from build123d import *

# Parameters (mm, degrees)
BOSS_EXTRUDE1_DEPTH = 6.5
SKETCH2_OUTSIDE_W   = 43.518
SKETCH2_OUTSIDE_H   = 43.054
SKETCH2_OUTSIDE_R   = 6.5
CUT_EXTRUDE1_DEPTH  = 6.5
CUT_EXTRUDE1_DRAFT  = -60
SKETCH3_OUTSIDE_W   = 43.518
SKETCH3_OUTSIDE_H   = 43.054
SKETCH3_OUTSIDE_R   = 6.5
CUT_EXTRUDE2_DEPTH  = 6.5
CUT_EXTRUDE2_DRAFT  = -60
SKETCH4_R           = 4.5
CUT_EXTRUDE3_DEPTH  = 13.125271319


with BuildPart() as part:
    # Sketch1 → Boss-Extrude1 (new body)
    with BuildSketch(Plane.XY):
        Polygon((4.981175881, 5.614376205), (-2.371604479, 7.121012956), (-7.352780361, 1.506636751), (-4.981175881, -5.614376205), (2.371604479, -7.121012956), (7.352780361, -1.506636751), align=None)
    extrude(amount=BOSS_EXTRUDE1_DEPTH)


with BuildPart() as cut_extrude1_tool:
    # Sketch2 outside → Cut-Extrude1 (with draft: the straight prism first)
    with BuildSketch(Plane.XY.offset(6.5)):
        Rectangle(SKETCH2_OUTSIDE_W, SKETCH2_OUTSIDE_H)
        Circle(SKETCH2_OUTSIDE_R, mode=Mode.SUBTRACT)
    extrude(amount=-CUT_EXTRUDE1_DEPTH)
    # Cut-Extrude1: the draft: its side faces are tilted about the plane it starts from
    cut_extrude1_sides = [cut_extrude1_tool.faces().sort_by_distance(p)[0] for p in [
        (0, -21.527, 3.25),
        (21.759, 0, 3.25),
        (0, 21.527, 3.25),
        (-21.759, 0, 3.25),
        (-6.5, 0, 3.25),
    ]]
    draft(cut_extrude1_sides, Plane.XY.offset(6.5), CUT_EXTRUDE1_DRAFT)


with BuildPart() as part_1:
    add(part.part)

    # Cut-Extrude1: cut by cut_extrude1_tool
    add(cut_extrude1_tool.part, mode=Mode.SUBTRACT)


with BuildPart() as cut_extrude2_tool:
    # Sketch3 outside → Cut-Extrude2 (with draft: the straight prism first)
    with BuildSketch(Plane(origin=(0, 0, 0), x_dir=(-1, 0, 0), z_dir=(0, 0, -1))):
        Rectangle(SKETCH3_OUTSIDE_W, SKETCH3_OUTSIDE_H)
        Circle(SKETCH3_OUTSIDE_R, mode=Mode.SUBTRACT)
    extrude(amount=-CUT_EXTRUDE2_DEPTH)
    # Cut-Extrude2: the draft: its side faces are tilted about the plane it starts from
    cut_extrude2_sides = [cut_extrude2_tool.faces().sort_by_distance(p)[0] for p in [
        (0, -21.527, 3.25),
        (-21.759, 0, 3.25),
        (0, 21.527, 3.25),
        (21.759, 0, 3.25),
        (6.5, 0, 3.25),
    ]]
    draft(cut_extrude2_sides, Plane(origin=(0, 0, 0), x_dir=(-1, 0, 0), z_dir=(0, 0, -1)), CUT_EXTRUDE2_DRAFT)


with BuildPart() as part_2:
    add(part_1.part)

    # Cut-Extrude2: cut by cut_extrude2_tool
    add(cut_extrude2_tool.part, mode=Mode.SUBTRACT)

    # Sketch4 → Cut-Extrude3 (cut, through all)
    with BuildSketch(Plane(origin=(0, 0, 0), x_dir=(-1, 0, 0), z_dir=(0, 0, -1))):
        Circle(SKETCH4_R)
    extrude(amount=-CUT_EXTRUDE3_DEPTH, mode=Mode.SUBTRACT)


solid = part_2.part
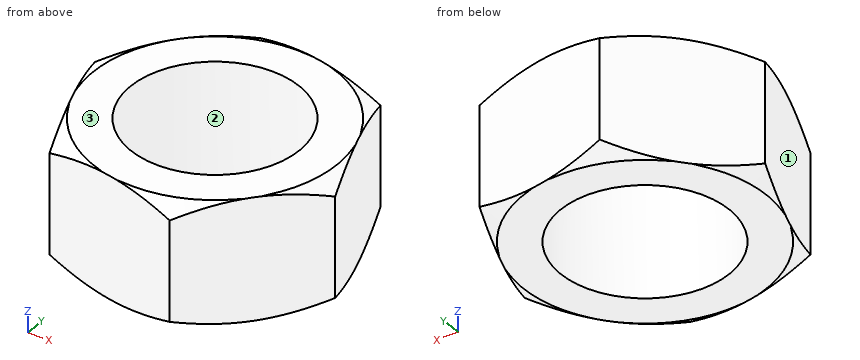
Design review of the part built by this model. Coordinates are the model's own, in mm. Face numbers are marked on the shaded views. Give positions to 0.01 mm unless a question says otherwise; leave off trailing zeros. Write each loop counter-clockwise with the first axis right and the second up, starting at its lowest first coordinate (ties: lowest second). Pieces come first, ordered by that corner, then holes. Notation, with made-up numbers: M 10,10.25 L 53,10.25 A24 cw 53,27.25 Z; hole C 22.5,13 d4. An arc over 180 degrees is marked long. Answer as a JSON object with one key per item and string values. Group by question number.
1) We need section B-B (x = 0). Give the boundary of the cut face in (y, z).
2) Clearance check with flat-ended pins moving along their axes: pin 1 Ø2 at (y, z) = (-1.5, 4.5) entering from -X; pin 2 Ø1.5 at (y, z) = (1, 5.5) entering from -X; pin 3 Ø1 at (x, z) = (4, 2) entering from +Y. State where each tip first meets the part, or that it passes through.
3) We need section A-A (z = 4). Give the boundary of the cut face in (x, y).
4) Mouldability with a two-part tool opening along Y and no side actions: class the marked faces 1, 2 and 3 as released by +Y, released by -Y, zero draft, split by the parting line, or undercut.
5) For line 1 along Y through (x, z) = (0, 4); line 2 along Y through (x, z) = (-3, 5); line 3 along X through (y, z) = (3.5, 1.75), list the stretches that pass through material, from the lowest coordinate up.
6) We need section C-C (y = 0). Give the boundary of the cut face in (x, z).
Answer key:
{
 "1": {"outline": "M -6.64,0.08 L -6.5,0 L -4.5,0 L -4.5,6.5 L -6.5,6.5 L -6.64,6.42 Z; M 4.5,0 L 6.5,0 L 6.64,0.08 L 6.64,6.42 L 6.5,6.5 L 4.5,6.5 Z"},
 "2": {"pin 1": "stops at x = -6.68", "pin 2": "stops at x = -7.35", "pin 3": "stops at y = 5.92"},
 "3": {"outline": "M -7.35,1.51 L -4.98,-5.61 L 2.37,-7.12 L 7.35,-1.51 L 4.98,5.61 L -2.37,7.12 Z; hole C 0,0 d9"},
 "4": {"face 1": "released by -Y", "face 2": "undercut", "face 3": "zero draft"},
 "5": {"line 1": "y = -6.64 to -4.5, 4.5 to 6.64", "line 2": "y = -6.02 to -3.35, 3.35 to 6.41", "line 3": "x = -5.58 to -2.83, 2.83 to 5.69"},
 "6": {"outline": "M -6.85,0.2 L -6.5,0 L -4.5,0 L -4.5,6.5 L -6.5,6.5 L -6.85,6.3 Z; M 4.5,0 L 6.5,0 L 6.85,0.2 L 6.85,6.3 L 6.5,6.5 L 4.5,6.5 Z"}
}
